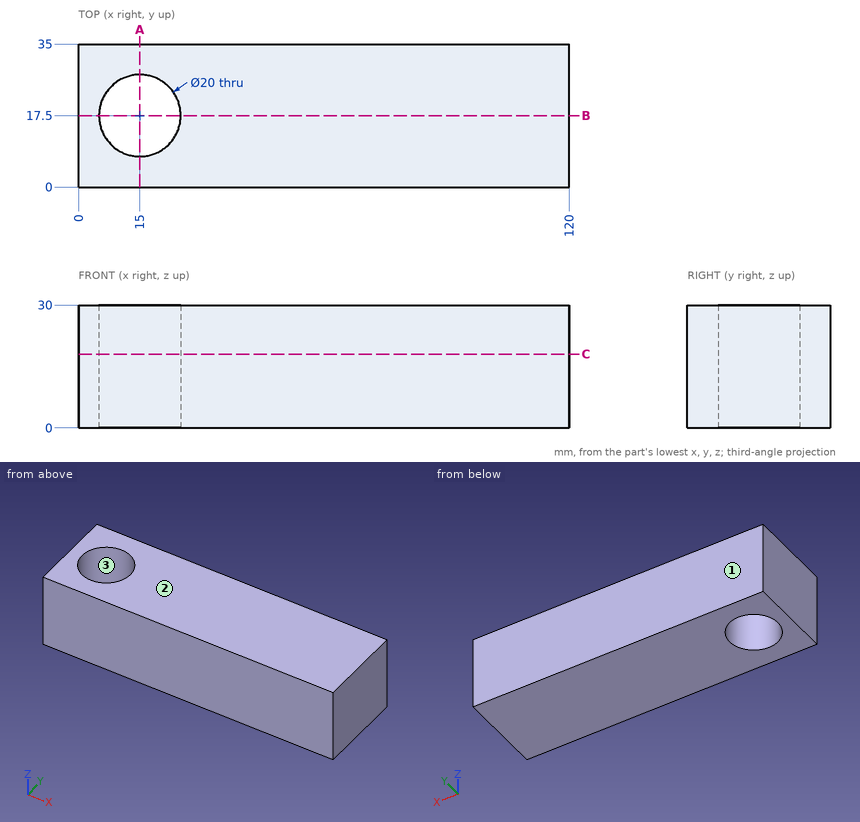
Geometry check sheet. Reference: drawing and pictorial views, mm from the part's lowest x, y, z. Round coordinates to 2 decimals unless told otherwise and drop trailing zeros. Loops run counter-clockwise (first coordinate to the right, second up) from the corner with the lowest first, then second, coordinate; pieces in that order, holes last. Notation, with made-up numbers: M -15.75,59.5 L 26.25,59.5 A10 cw 26.25,74.5 Z; hole C -7.75,-10.75 d4. An arc over 180 degrees is marked long. Return JSON: item names as keys, results as strings. Group by question number.
(1) Scan lines: line 1 along Y through (x, z) = (15, 13); line 2 along X through (y, z) = (26, 16.25); line 3 along X through (y, z) = (25, 12.75). Record each from-to range of solid material in increasing order. Write a range as [from, to].
(2) Mould release check, pull along Y, two halves, no side actions. Record for the marked faces 1, 2 and 3: pulls with the +Y half, pulls with the -Y half, needs draft (parallel to the pull), parting line crosses it, or undercut.
(3) Section check B-B, the plane y = 17.5. Enter the section's corners in (x, z).
(4) Section check C-C, the plane z = 18. Enter the section's corners in (x, y).
(5) Section check A-A, the plane x = 15. Enter the section's corners in (y, z), and give its area (3 significant figures).
Data:
{
 "1": {"line 1": "[0, 7.5], [27.5, 35]", "line 2": "[0, 9.73], [20.27, 120]", "line 3": "[0, 8.39], [21.61, 120]"},
 "2": {"face 1": "pulls with the +Y half", "face 2": "needs draft", "face 3": "undercut"},
 "3": {"outline": "M 0,0 L 5,0 L 5,30 L 0,30 Z; M 25,0 L 120,0 L 120,30 L 25,30 Z"},
 "4": {"outline": "M 0,0 L 120,0 L 120,35 L 0,35 Z; hole C 15,17.5 d20"},
 "5": {"outline": "M 0,0 L 7.5,0 L 7.5,30 L 0,30 Z; M 27.5,0 L 35,0 L 35,30 L 27.5,30 Z", "area": "450 mm²"}
}
